Source: CAD feature listing. Evaluate the final solid. Frame: model axes, mm. Round coordinates to 2 decimals unless told otherwise and drop trailing zeros. Write each loop counter-clockwise with the first axis right and the second up, starting at its lowest first coordinate (ties: lowest second). Pieces come first, ordered by that corner, then holes.
from build123d import *

# Parameters (mm, degrees)
CROQUIS1_W              = 100
CROQUIS1_H              = 116
CROQUIS1_R              = 1.5
SALIENTE_EXTRUIR1_DEPTH = 15
CROQUIS3_R              = 11
CORTAR_EXTRUIR2_DEPTH   = 7


with BuildPart() as part:
    # Croquis1 → Saliente-Extruir1 (new body)
    with BuildSketch(Plane(origin=(0, 0, 0), x_dir=(0, 0, -1), z_dir=(1, 0, 0))):
        with Locations((50, 58)):
            Rectangle(CROQUIS1_W, CROQUIS1_H)
        with Locations((5, 110)):
            Circle(CROQUIS1_R, mode=Mode.SUBTRACT)
        with Locations((29, 110)):
            Circle(CROQUIS1_R, mode=Mode.SUBTRACT)
        with Locations((5, 92)):
            Circle(CROQUIS1_R, mode=Mode.SUBTRACT)
        with Locations((29, 92)):
            Circle(CROQUIS1_R, mode=Mode.SUBTRACT)
        with Locations(Location((5, 24, 0), (0, 0, 180))):
            Circle(CROQUIS1_R, mode=Mode.SUBTRACT)
        with Locations(Location((29, 24, 0), (0, 0, 180))):
            Circle(CROQUIS1_R, mode=Mode.SUBTRACT)
        with Locations(Location((29, 6, 0), (0, 0, 180))):
            Circle(CROQUIS1_R, mode=Mode.SUBTRACT)
        with Locations(Location((5, 6, 0), (0, 0, 180))):
            Circle(CROQUIS1_R, mode=Mode.SUBTRACT)
        with Locations((31.2, 58)):
            Circle(CROQUIS1_R, mode=Mode.SUBTRACT)
        with Locations((68.8, 58)):
            Circle(CROQUIS1_R, mode=Mode.SUBTRACT)
        with Locations((71, 6)):
            Circle(CROQUIS1_R, mode=Mode.SUBTRACT)
        with Locations((95, 6)):
            Circle(CROQUIS1_R, mode=Mode.SUBTRACT)
        with Locations((95, 24)):
            Circle(CROQUIS1_R, mode=Mode.SUBTRACT)
        with Locations((71, 24)):
            Circle(CROQUIS1_R, mode=Mode.SUBTRACT)
        with Locations(Location((95, 92, 0), (0, 0, 180))):
            Circle(CROQUIS1_R, mode=Mode.SUBTRACT)
        with Locations(Location((71, 92, 0), (0, 0, 180))):
            Circle(CROQUIS1_R, mode=Mode.SUBTRACT)
        with Locations(Location((71, 110, 0), (0, 0, 180))):
            Circle(CROQUIS1_R, mode=Mode.SUBTRACT)
        with Locations(Location((95, 110, 0), (0, 0, 180))):
            Circle(CROQUIS1_R, mode=Mode.SUBTRACT)
    extrude(amount=SALIENTE_EXTRUIR1_DEPTH)

    # Croquis3 → Cortar-Extruir2 (cut)
    with BuildSketch(Plane.ZY):
        with Locations((-46.5, 99)):
            Circle(CROQUIS3_R)
        with Locations((-46.5, 17)):
            Circle(CROQUIS3_R)
    extrude(amount=-CORTAR_EXTRUIR2_DEPTH, mode=Mode.SUBTRACT)


solid = part.part
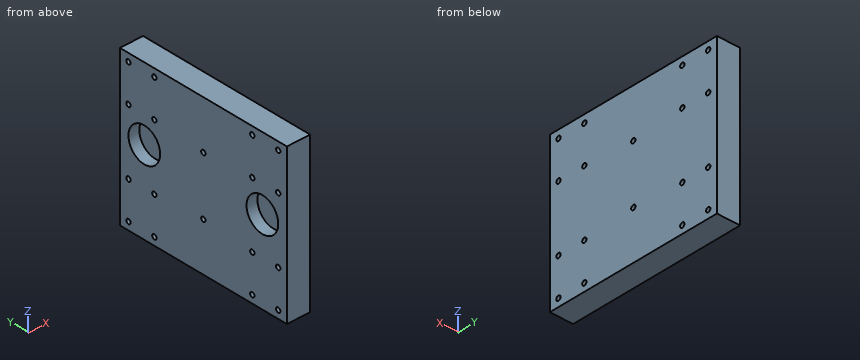
1) Section query C-C on z = -95. Return the cut outline in (x, y), then the cut area to 3 significant figures.
Taken from the geometry:
outline: (0, 0) - (15, 0) - (15, 4.5) - (0, 4.5) - close; (0, 7.5) - (15, 7.5) - (15, 22.5) - (0, 22.5) - close; (0, 25.5) - (15, 25.5) - (15, 90.5) - (0, 90.5) - close; (0, 93.5) - (15, 93.5) - (15, 108.5) - (0, 108.5) - close; (0, 111.5) - (15, 111.5) - (15, 116) - (0, 116) - close
area: 1,560 mm2
2) Section query B-B on y = 58. Return the cut outline in (x, z).
Taken from the geometry:
outline: (0, -100) - (15, -100) - (15, -70.3) - (0, -70.3) - close; (0, -67.3) - (15, -67.3) - (15, -32.7) - (0, -32.7) - close; (0, -29.7) - (15, -29.7) - (15, 0) - (0, 0) - close
3) Section query D-D on y = 92. Return the cut outline in (x, z).
Taken from the geometry:
outline: (0, -100) - (15, -100) - (15, -96.5) - (0, -96.5) - close; (0, -93.5) - (15, -93.5) - (15, -72.5) - (0, -72.5) - close; (0, -69.5) - (15, -69.5) - (15, -30.5) - (0, -30.5) - (0, -38.01) - (7, -38.01) - (7, -54.99) - (0, -54.99) - close; (0, -27.5) - (15, -27.5) - (15, -6.5) - (0, -6.5) - close; (0, -3.5) - (15, -3.5) - (15, 0) - (0, 0) - close
4) Material intervals for line 1 (Y direction, x = 9, z = -5); line 2 (Y direction, x = 2, z = -46.5); line 3 (Y direction, x = 9.75, z = -68.8), sorted ascending.
Taken from the geometry:
line 1: y = 0 to 4.5, 7.5 to 22.5, 25.5 to 90.5, 93.5 to 108.5, 111.5 to 116
line 2: y = 0 to 6, 28 to 88, 110 to 116
line 3: y = 0 to 56.5, 59.5 to 116
5) Section query A-A on x = 2.25. State how many separate pieces and enclosed holes the cut face has, then the cut area to 3 significant figures.
Taken from the geometry:
separate pieces: 1
enclosed holes: 20
area: 10,700 mm2
6) Contact query for flat-ended pins moving along their axis: P1, Ø2.5, axis at y = 110, z = -29, coming from the +X side; P2, Ø4, axis at y = 110, z = -71, coming from the -X side. Output: stop coordinate, or through.
Taken from the geometry:
P1: passes through
P2: stops at x = 0
